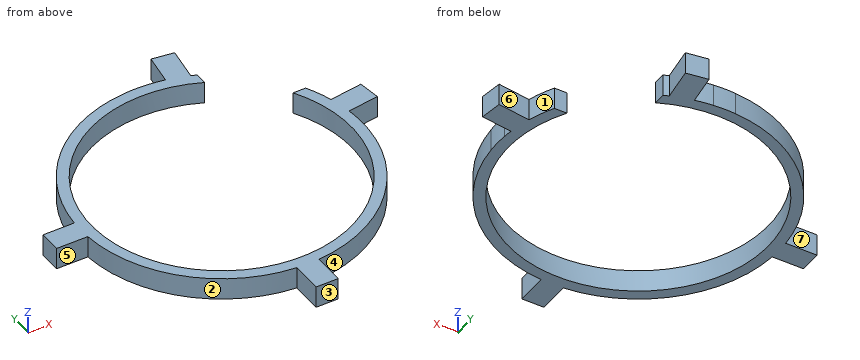
Autodesk Inventor part; units mm, degrees
ref_plane "YZ Plane" through (0, 0, 0) normal (1, 0, 0) x (0, 1, 0)
ref_plane "XZ Plane" through (0, 0, 0) normal (0, 1, 0) x (-1, 0, 0)
ref_plane "XY Plane" through (0, 0, 0) normal (0, 0, 1) x (1, 0, 0)
sketch "Sketch1" plane through (0, 0, 0) normal (0, 0, 1) x (1, 0, 0)
  arc A0 (-25.4018, 15) -> (25.4018, 15) centre (0, 0) ccw
  line L0 (25.4018, 15) -> (28.2666, 15)
  line L1 (-39, 2.5) -> (-32, 2.5)
  line L2 (-32, -2.5) -> (-39, -2.5)
  line L3 (-39, -2.5) -> (-39, 2.5)
  line L4 (-32, 2.5) -> (-31.9022, 2.5)
  line L5 (-32, -2.5) -> (-31.9022, -2.5)
  line L6 (2.5, -32) -> (2.5, -39)
  line L7 (2.5, -39) -> (-2.5, -39)
  line L8 (-2.5, -39) -> (-2.5, -32)
  line L9 (-2.5, -32) -> (-2.5, -31.9022)
  line L10 (2.5, -32) -> (2.5, -31.9022)
  arc A1 (-28.2666, 15) -> (-31.9022, 2.5) centre (0, 0) ccw
  arc A2 (-31.9022, -2.5) -> (-2.5, -31.9022) centre (0, 0) ccw
  arc A3 (2.5, -31.9022) -> (31.9022, -2.5) centre (0, 0) ccw
  arc A4 (12.5, 26.7208) -> (25.4018, 15) centre (0, 0) ccw
  line L11 (12.5, 29.4576) -> (12.5, 26.7208)
  arc A5 (-2.5, 31.9022) -> (-31.9022, 2.5) centre (0, 0) ccw
  arc A6 (-31.9022, -2.5) -> (-2.5, -31.9022) centre (0, 0) ccw
  arc A7 (2.5, -31.9022) -> (31.9022, -2.5) centre (0, 0) ccw
  line L12 (6.5, 31.3329) -> (7.5001, 38.3601)
  line L13 (6.5, 31.3329) -> (13.598, 31.3329) construction
  line L14 (7.5001, 38.3601) -> (12.4502, 37.6556)
  line L15 (12.4502, 37.6556) -> (11.3493, 29.9198)
  arc A8 (12.5, 29.4576) -> (11.3493, 29.9198) centre (0, 0) ccw
  arc A9 (12.5, 29.4576) -> (11.3493, 29.9198) centre (0, 0) ccw
  arc A10 (6.5, 31.3329) -> (2.5, 31.9022) centre (0, 0) ccw
  arc A11 (6.5, 31.3329) -> (-31.9022, 2.5) centre (0, 0) ccw
  arc A12 (-31.9022, -2.5) -> (-2.5, -31.9022) centre (0, 0) ccw
  arc A13 (2.5, -31.9022) -> (31.9022, -2.5) centre (0, 0) ccw
  line L16 (31.682, 4.5) -> (32.601, 4.5) construction
  line L17 (31.682, 4.5) -> (39.0737, 4.5) construction
  line L18 (-2.5, 31.9022) -> (4.598, 31.9022) construction
  line L19 (31.682, 4.5) -> (38.7092, 5.5001)
  line L20 (31.682, 4.5) -> (38.78, 4.5) construction
  line L21 (38.7092, 5.5001) -> (38.0047, 10.4502)
  line L22 (38.0047, 10.4502) -> (30.5898, 9.3949)
  arc A14 (30.5898, 9.3949) -> (28.2666, 15) centre (0, 0) ccw
  arc A15 (31.9022, 2.5) -> (31.682, 4.5) centre (0, 0) ccw
  arc A16 (30.5898, 9.3949) -> (28.2666, 15) centre (0, 0) ccw
  arc A17 (31.9022, 2.5) -> (31.682, 4.5) centre (0, 0) ccw
  arc A18 (30.5898, 9.3949) -> (28.2666, 15) centre (0, 0) ccw
  arc A19 (31.9022, 2.5) -> (31.682, 4.5) centre (0, 0) ccw
  arc A20 (30.5898, 9.3949) -> (28.2666, 15) centre (0, 0) ccw
  arc A21 (12.5, 29.4576) -> (11.3493, 29.9198) centre (0, 0) ccw
  arc A22 (2.5, -31.9022) -> (31.682, 4.5) centre (0, 0) ccw
  arc A23 (6.5, 31.3329) -> (-31.9022, 2.5) centre (0, 0) ccw
  arc A24 (-31.9022, -2.5) -> (-2.5, -31.9022) centre (0, 0) ccw
  point P0 (11.5, 29.8622)
  point P1 (2.5, 31.9022)
  point P2 (31.9022, -2.5)
  dimension "d78" = 7.098
  dimension "d79" = 81.9
  dimension "d80" = 5
  dimension "d81" = 90
  dimension "d82" = 90
  dimension "d94" = 7.098
  dimension "d95" = 8.1
  dimension "d96" = 5
  dimension "d97" = 90
  dimension "d98" = 90
extrude "Extrusion7" add sketch "Sketch1" along normal blind 5
properties part number "Clip_TestFitV1"
For this review, take the finished solid that the model builds, in its own axes (mm). Face numbers are marked on the shaded views. A direction names the side the tool comes from. Give positions to 0.01 mm unless a question says otherwise; leave off trailing zeros. Write each loop counter-clockwise with the first axis right and the second up, starting at its lowest first coordinate (ties: lowest second). Pieces come first, ordered by that corner, then holes. Notation, with made-up numbers: (75, 89.5) -> (107, 89.5) arc R30 ccw to (107, 121.5) -> close; hole circle Ø10 at (65.5, -21). An arc over 180 degrees is marked (long way). Use CSV: the item, a comma, the result in double quotes.
Q1. Take a section at D-D, the plane x = 17.5. Write out the cut boundary in (y, z), then the cut area to 3 significant figures.
Conclusion:
outline,"(-26.79, 0) -> (-23.75, 0) -> (-23.75, 5) -> (-26.79, 5) -> close"
area,"15.2 mm2"
Q2. Mouldability with a two-part tool opening along X and no side actions: class the marked faces 1, 2, 3 and 4 as pulls with the +X half, pulls with the -X half, needs draft (parallel to the pull), parting line crosses it, or undercut.
Conclusion:
face 1,"undercut"
face 2,"pulls with the -X half"
face 3,"needs draft"
face 4,"pulls with the +X half"
Q3. Take a section at A-A, the plane y = -15. Write out the cut boundary in (x, z).
Conclusion:
outline,"(-28.27, 0) -> (-25.4, 0) -> (-25.4, 5) -> (-28.27, 5) -> close; (25.4, 0) -> (28.27, 0) -> (28.27, 5) -> (25.4, 5) -> close"
Q4. To check wall thickness, follow probe 1 along X at (y, z) = (0, 3.5); probe 2 along X at (y, z) = (-4.5, 4.5). State the ranges of each line that lie inside material, in increasing order. Write a range as [from, to].
Conclusion:
probe 1,"[-39, -29.5], [29.5, 32]"
probe 2,"[-31.68, -29.15], [29.15, 31.68]"
Q5. Tool access review of the marked faces 5, 6 and 7: name each direction out of +Z, -Z, +X, -X, +Y, -Y from which nothing blocks a thin tool from reaching the whole face with its end or side.
Conclusion:
face 5,"+Z, -Z, -X, -Y"
face 6,"+Z, -Z, +Y"
face 7,"+Z, -Z, -X, +Y"
Q6. For P1, Ø1.4, axis at y = 28.5, z = 1.5, coming from the +X side; P2, Ø1.5, axis at x = -28, y = 3, coming from the -Z side; P3, Ø1, axis at y = -21, z = 0.5, coming from the -X side; P4, Ø1, axis at x = 9, z = 3, coming from the +Y side, all flat-tipped, find the tip position at first contact; note any pin that passes through.
Conclusion:
P1,"x = 12.5"
P2,"through"
P3,"x = -24.57"
P4,"y = 38.22"
Q7. Take a section at C-C, the plane z = 1.3. Write out the cut boundary in (x, y).
Conclusion:
outline,"(-39, -2.5) -> (-31.9, -2.5) arc R32 ccw to (-2.5, -31.9) -> (-2.5, -39) -> (2.5, -39) -> (2.5, -31.9) arc R32 ccw to (31.9, -2.5) arc R32 ccw to (31.9, 2.5) arc R31.98 ccw to (31.68, 4.5) -> (38.71, 5.5) -> (38, 10.45) -> (30.59, 9.39) arc R32 ccw to (28.27, 15) -> (25.4, 15) arc R29.5 cw (long way) to (-25.4, 15) arc R29.5 cw to (12.5, 26.72) -> (12.5, 29.46) arc R32.04 ccw to (11.35, 29.92) -> (12.45, 37.66) -> (7.5, 38.36) -> (6.5, 31.33) arc R32 ccw to (2.5, 31.9) arc R32 ccw to (-2.5, 31.9) arc R32 ccw to (-28.27, 15) arc R32 ccw to (-31.9, 2.5) -> (-39, 2.5) -> close"
Q8. Take a section at B-B, the plane x = 0. Write out the cut boundary in (y, z), then the cut area to 3 significant figures.
Conclusion:
outline,"(-39, 0) -> (-29.5, 0) -> (-29.5, 5) -> (-39, 5) -> close; (29.5, 0) -> (32, 0) -> (32, 5) -> (29.5, 5) -> close"
area,"60.0 mm2"
